Read the model definition and answer for the solid it produces. Units are mm, in the model's axes. A direction names the side the tool comes from. Give positions to 0.01 mm unless a question says otherwise; leave off trailing zeros. Write each loop counter-clockwise with the first axis right and the second up, starting at its lowest first coordinate (ties: lowest second). Pieces come first, ordered by that corner, then holes.
```python
from build123d import *

# Parameters (mm, degrees)
BOSS_EXTRUDE1_DEPTH = 100
CUT_EXTRUDE1_DEPTH  = 70
SKETCH3_W           = 55
SKETCH3_H           = 70
CUT_EXTRUDE2_DEPTH  = 70
FILLET1_R           = 25
CUT_EXTRUDE3_REACH  = 214.047
SKETCH4_R           = 17
CUT_EXTRUDE4_DEPTH  = 25
CUT_EXTRUDE5_START  = -25
CUT_EXTRUDE5_DEPTH  = 25
CUT_EXTRUDE6_DEPTH  = 85


with BuildPart() as part:
    # Sketch1 → Boss-Extrude1 (new body)
    with BuildSketch(Plane(origin=(0, 0, 0), x_dir=(1, 0, 0), z_dir=(0, 1, 0))):
        with BuildLine():
            Line((0, 5), (0, 115))
            ThreePointArc((0, 115), (1.464466094, 118.535533906), (5, 120))
            Line((5, 120), (25, 120))
            ThreePointArc((25, 120), (28.535533906, 121.464466094), (30, 125))
            Line((30, 125), (30, 153))
            ThreePointArc((30, 153), (31.464466094, 156.535533906), (35, 158))
            Line((35, 158), (68, 158))
            Line((68, 158), (110.425847486, 118.437257177))
            ThreePointArc((110.425847486, 118.437257177), (132.286586918, 87.505026337), (140, 50.421362927))
            Line((140, 50.421362927), (140, -50))
            Line((140, -50), (125, -50))
            ThreePointArc((125, -50), (121.464466094, -51.464466094), (120, -55))
            Line((120, -55), (120, -70))
            Line((120, -70), (40, -70))
            Line((40, -70), (40, -5))
            ThreePointArc((40, -5), (38.535533906, -1.464466094), (35, 0))
            Line((35, 0), (5, 0))
            ThreePointArc((5, 0), (1.464466094, 1.464466094), (0, 5))
        make_face()
    extrude(amount=BOSS_EXTRUDE1_DEPTH)

    # Sketch2 → Cut-Extrude1 (cut)
    with BuildSketch(Plane(origin=(0, 15, 0), x_dir=(-1, 0, 0), z_dir=(0, -1, 0))):
        with BuildLine():
            Line((-53.337208144, 158), (-103.605863885, 111.123720161))
            ThreePointArc((-103.605863885, 111.123720161), (-123.115986174, 83.517535648), (-130, 50.421362927))
            Line((-130, 50.421362927), (-130, -50))
            Line((-130, -50), (-140, -50))
            Line((-140, -50), (-140, 50.421362927))
            ThreePointArc((-140, 50.421362927), (-132.286586918, 87.505026337), (-110.425847486, 118.437257177))
            Line((-110.425847486, 118.437257177), (-68, 158))
            Line((-68, 158), (-53.337208144, 158))
        make_face()
    extrude(amount=-CUT_EXTRUDE1_DEPTH, mode=Mode.SUBTRACT)

    # Sketch3 → Cut-Extrude2 (cut)
    with BuildSketch(Plane(origin=(0, 100, 0), x_dir=(1, 0, 0), z_dir=(0, 1, 0))):
        with Locations((112.5, -35)):
            Rectangle(SKETCH3_W, SKETCH3_H)
    extrude(amount=-CUT_EXTRUDE2_DEPTH, mode=Mode.SUBTRACT)

    # Fillet1
    fillet1_edges = [part.edges().sort_by_distance(p)[0] for p in [
        (62.5, 100, 70),
    ]]
    fillet(fillet1_edges, radius=FILLET1_R)

    # Sketch4 → Cut-Extrude3 (cut, up to next)
    with BuildSketch(Plane.ZY.offset(-40), mode=Mode.PRIVATE) as cut_extrude3_sk1:
        with Locations((35, 65)):
            Circle(SKETCH4_R)
    cut_extrude3_tool1 = extrude(cut_extrude3_sk1.sketch, amount=-CUT_EXTRUDE3_REACH, mode=Mode.PRIVATE) & part.part
    add(cut_extrude3_tool1.solids().sort_by_distance((40, 65, 35))[0], mode=Mode.SUBTRACT)

    # Sketch5 → Cut-Extrude4 (cut)
    with BuildSketch(Plane(origin=(0, 100, 0), x_dir=(1, 0, 0), z_dir=(0, 1, 0))):
        with BuildLine():
            Line((30, 90), (30, 33))
            ThreePointArc((30, 33), (20, 23), (10, 33))
            Line((10, 33), (10, 90))
            ThreePointArc((10, 90), (20, 100), (30, 90))
        make_face()
    extrude(amount=-CUT_EXTRUDE4_DEPTH, mode=Mode.SUBTRACT)

    # Sketch6 → Cut-Extrude5 (cut)
    with BuildSketch(Plane.XZ.offset(CUT_EXTRUDE5_START)):
        with BuildLine():
            Line((30, -33), (30, -90))
            ThreePointArc((30, -90), (20, -100), (10, -90))
            Line((10, -90), (10, -33))
            ThreePointArc((10, -33), (20, -23), (30, -33))
        make_face()
    extrude(amount=CUT_EXTRUDE5_DEPTH, mode=Mode.SUBTRACT)

    # Sketch7 → Cut-Extrude6 (cut)
    with BuildSketch(Plane(origin=(0, 100, 0), x_dir=(1, 0, 0), z_dir=(0, 1, 0))):
        with BuildLine():
            Line((55, 115), (55, 43))
            ThreePointArc((55, 43), (56.464466094, 39.464466094), (60, 38))
            Line((60, 38), (121, 38))
            ThreePointArc((121, 38), (124.535533906, 39.464466094), (126, 43))
            Line((126, 43), (126, 55))
            ThreePointArc((126, 55), (114.251031375, 92.577557769), (86, 120))
            Line((86, 120), (60, 120))
            ThreePointArc((60, 120), (56.464466094, 118.535533906), (55, 115))
        make_face()
    extrude(amount=-CUT_EXTRUDE6_DEPTH, mode=Mode.SUBTRACT)


solid = part.part
```
Item 1: Section A-A (y = 57) is taken. Give the number of separate pieces and of enclosed holes in the cut face, and give its area (3 significant figures).
Result set:
separate pieces: 2
enclosed holes: 1
area: 13,300 mm2
Item 2: Which of the six approach directions +Z, -Z, +X, -X, +Y, -Y give full straight-line access (tool end or side, diameter ignored) to faces 5 (the cylindrical face through (122.925, 49.51, -83.954)), 6 (the flat face through (20, 25, -61)), 7 (the flat face through (126, 58, -49)), 8 (the flat face through (106, 65, 0))?
Result set:
face 5: -Z, +X
face 6: -Y
face 7: +Y
face 8: +Z, +X, +Y
Item 3: Find the intervals of material crossed by line 1 along X through (y, z) = (89, -45); line 2 along Y through (x, z) = (68, 35); line 3 along X through (y, z) = (53, 9), in increasing order.
Result set:
line 1: x = 0 to 10, 30 to 55, 126 to 140
line 2: y = 0 to 48, 82 to 100
line 3: x = 40 to 85
Item 4: Section B-B (z = 35) is taken. Write down the section's boundary in (x, y).
Result set:
outline: (40, 0) - (140, 0) - (140, 15) - (130, 15) - (130, 30) - (85, 30) - (85, 48) - (40, 48) - close; (40, 82) - (85, 82) - (85, 100) - (40, 100) - close
Item 5: Each of these flat-tipped pins is pushed along its axis until it touches: pin 1 Ø1 at (y, z) = (71.5, -63.5) entering from +X; pin 2 Ø3 at (y, z) = (34.5, 17) entering from +X; pin 3 Ø12 at (x, z) = (96, -109) entering from +Y; pin 4 Ø3 at (y, z) = (50.5, -33.5) entering from +X. Where does it stop, or does it pass through?
Result set:
pin 1: stops at x = 129.04
pin 2: stops at x = 85
pin 3: stops at y = 100
pin 4: stops at x = 130
Item 6: Section C-C (x = 20) is taken. Write down the section's boundary in (y, z).
Result set:
outline: (0, -120) - (100, -120) - (100, -100) - (75, -100) - (75, -23) - (100, -23) - (100, 0) - (0, 0) - (0, -23) - (25, -23) - (25, -100) - (0, -100) - close
Item 7: Determine the mould class of faces 1 (the cylindrical face through (62.185, 92.871, 62.482)), 2 (the flat face through (85, 49.9, 43.3)), 3 (the flat face through (10, 13, -62)), 4 (the flat face through (40, 49, 45)) for opening direction X: pulls with the +X half, pulls with the -X half, needs draft (parallel to the pull), parting line crosses it, or undercut.
Result set:
face 1: needs draft
face 2: pulls with the +X half
face 3: undercut
face 4: pulls with the -X half
